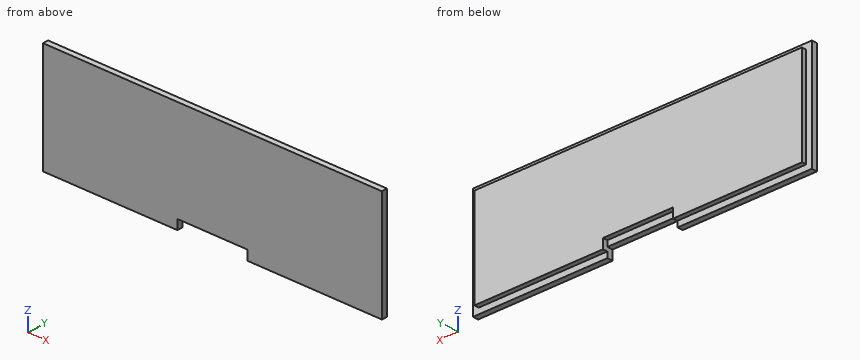
from build123d import *

# Parameters (mm, degrees)
SKICA1_W                 = 72.4
SKICA1_H                 = 22.9
P_IDAT_VYSUNUT_M2_DEPTH  = 1.2
SKICA2_W                 = 70
SKICA2_H                 = 20.5
P_IDAT_VYSUNUT_M3_DEPTH  = 1
SKICA3_W                 = 15
SKICA3_H                 = 2
ODEBRAT_VYSUNUT_M1_DEPTH = 10
SKICA4_W                 = 15
SKICA4_H                 = 1.2
ODEBRAT_VYSUNUT_M2_DEPTH = 1


with BuildPart() as part:
    # Skica1 → Přidat vysunutím2 (new body)
    with BuildSketch(Plane(origin=(0, 0, 0), x_dir=(1, 0, 0), z_dir=(0, 1, 0))):
        with Locations((36.2, 11.45)):
            Rectangle(SKICA1_W, SKICA1_H)
    extrude(amount=P_IDAT_VYSUNUT_M2_DEPTH)

    # Skica2 → Přidat vysunutím3 (add)
    with BuildSketch(Plane(origin=(0, 1.2, 0), x_dir=(1, 0, 0), z_dir=(0, 1, 0))):
        with Locations((36.2, 11.45)):
            Rectangle(SKICA2_W, SKICA2_H)
    extrude(amount=P_IDAT_VYSUNUT_M3_DEPTH)

    # Skica3 → Odebrat vysunutím1 (cut)
    with BuildSketch(Plane(origin=(0, 2.2, 0), x_dir=(1, 0, 0), z_dir=(0, 1, 0))):
        with Locations((36.2, 21.9)):
            Rectangle(SKICA3_W, SKICA3_H)
    extrude(amount=-ODEBRAT_VYSUNUT_M1_DEPTH, mode=Mode.SUBTRACT)

    # Skica4 → Odebrat vysunutím2 (cut)
    with BuildSketch(Plane(origin=(0, 2.2, 0), x_dir=(1, 0, 0), z_dir=(0, 1, 0))):
        with Locations((36.2, 20.3)):
            Rectangle(SKICA4_W, SKICA4_H)
    extrude(amount=-ODEBRAT_VYSUNUT_M2_DEPTH, mode=Mode.SUBTRACT)


solid = part.part
The model under review builds one solid part; all positions refer to its coordinate system, in mm. Round coordinates to 2 decimals unless told otherwise and drop trailing zeros. Loops run counter-clockwise (first coordinate to the right, second up) from the corner with the lowest first, then second, coordinate; pieces in that order, holes last. Notation, with made-up numbers: M 18,29.25 L 26,29.25 A32 ccw 26,61.25 Z; hole C 89.5,78.5 d2. An arc over 180 degrees is marked long. Answer as a JSON object with one key per item and string values.
Item 1: Clearance check with flat-ended pins moving along their axes: P1, Ø1.1, axis at x = 38.5, y = 1.5, coming from the -Z side; P2, Ø1, axis at x = 36.5, z = -20, coming from the +Y side; P3, Ø1.1, axis at x = 48.5, y = 2, coming from the +Z side; P4, Ø0.5, axis at y = 1.5, z = -14.5, coming from the -X side. State where each tip first meets the part, or that it passes through.
Check sheet entries:
{"P1": "z = -20.9", "P2": "y = 2.2", "P3": "z = -1.2", "P4": "x = 1.2"}
Item 2: We need section B-B, the plane z = -14. State the section outline as (x, y) points.
Check sheet entries:
{"outline": "M 0,0 L 72.4,0 L 72.4,1.2 L 71.2,1.2 L 71.2,2.2 L 1.2,2.2 L 1.2,1.2 L 0,1.2 Z"}
Item 3: For line 1 along X through (y, z) = (0.7, -21.5); line 2 along Z through (x, y) = (45, 1.85); line 3 along X through (y, z) = (1.3, -7.25), list the stretches that pass through material, from the lowest coordinate up.
Check sheet entries:
{"line 1": "0 to 28.7, 43.7 to 72.4", "line 2": "-21.7 to -1.2", "line 3": "1.2 to 71.2"}
Item 4: We need section A-A, the plane x = 36. State the section outline as (y, z) points, and give its area (3 significant figures).
Check sheet entries:
{"outline": "M 0,-20.9 L 1.2,-20.9 L 1.2,-19.7 L 2.2,-19.7 L 2.2,-1.2 L 1.2,-1.2 L 1.2,0 L 0,0 Z", "area": "43.6 mm2"}
